from build123d import *

# Parameters (mm, degrees)
SKETCH_2_W               = 12.1
SKETCH_2_H               = 8
EXTRUDE_1_DEPTH          = 12.4
CUT_EXTRUDE_1_DEPTH      = 12.1
CUT_EXTRUDE_2_DEPTH      = 23.1
CUT_EXTRUDE_2_DEPTH_BACK = 16.1
HOLE_WIZARD_M31_D        = 3.4
HOLE_WIZARD_M31_DEPTH    = 10
HOLE_WIZARD_M31_TIP      = 1.021463052
FILLET_1_R               = 1


with BuildPart() as part:
    # Эскиз2 → Бобышка-Вытянуть1 (new body)
    with BuildSketch(Plane(origin=(0, 0, 0), x_dir=(0, 0, -1), z_dir=(1, 0, 0))):
        Polygon((-20.1, 10), (-20.1, 7), (0, 7), (0, 10), (15.1, 10), (15.1, -20), (12.1, -20), (12.1, 0), (0, 0), (0, -20), (-3, -20), (-3, 0), (-22.1, 0), (-22.1, 10), align=None)
        with Locations((6.05, -4)):
            Rectangle(SKETCH_2_W, SKETCH_2_H)
    extrude(amount=EXTRUDE_1_DEPTH)

    # Эскиз3 → Вырез-Вытянуть1 (cut)
    with BuildSketch(Plane.XY):
        with BuildLine():
            Line((0, 0), (-4.310236897, 0))
            Line((-4.310236897, 0), (-4.310236897, -10.158248203))
            Line((-4.310236897, -10.158248203), (16.784307367, -10.158248203))
            Line((16.784307367, -10.158248203), (16.784307367, 0))
            Line((16.784307367, 0), (12.4, 0))
            ThreePointArc((12.4, 0), (6.2, -6.2), (0, 0))
        make_face()
    extrude(amount=-CUT_EXTRUDE_1_DEPTH, mode=Mode.SUBTRACT)

    # Эскиз4 → Вырез-Вытянуть2 (cut, two sides)
    with BuildSketch(Plane.XY) as cut_extrude_2_sk:
        with BuildLine():
            Line((0, -13.8), (-4.529189241, -13.8))
            Line((-4.529189241, -13.8), (-4.529189241, -23.032738442))
            Line((-4.529189241, -23.032738442), (17.457291493, -23.032738442))
            Line((17.457291493, -23.032738442), (17.457291493, -13.8))
            Line((17.457291493, -13.8), (12.4, -13.8))
            ThreePointArc((12.4, -13.8), (6.2, -20), (0, -13.8))
        make_face()
    extrude(amount=CUT_EXTRUDE_2_DEPTH, mode=Mode.SUBTRACT)
    extrude(cut_extrude_2_sk.sketch, amount=-CUT_EXTRUDE_2_DEPTH_BACK, mode=Mode.SUBTRACT)

    # Отверстие с зазором M31
    with Locations(Plane(origin=(0, 7, 0), x_dir=(1, 0, 0), z_dir=(0, 1, 0))):
        with Locations((6.25, -10.05)):
            Hole(HOLE_WIZARD_M31_D / 2, depth=HOLE_WIZARD_M31_DEPTH)
            with Locations((0, 0, -(HOLE_WIZARD_M31_DEPTH + HOLE_WIZARD_M31_TIP / 2))):  # 118° drill point
                Cone(0, HOLE_WIZARD_M31_D / 2, HOLE_WIZARD_M31_TIP, mode=Mode.SUBTRACT)

    # Скругление1
    fillet_1_edges = [part.edges().sort_by_distance(p)[0] for p in [
        (6.2, 0, 22.1),
        (6.2, 10, 22.1),
    ]]
    fillet(fillet_1_edges, radius=FILLET_1_R)

    # Эскиз9 → Повернуть1 (revolve)
    with BuildSketch(Plane(origin=(6.2, 0, 0), x_dir=(0, 0, -1), z_dir=(1, 0, 0))):
        with BuildLine():
            Line((12.1, -20), (12.1, -18))
            Line((12.1, -18), (11.3, -18))
            ThreePointArc((11.3, -18), (11.507417596, -19.077032961), (12.1, -20))
        make_face()
    revolve(axis=Axis((6.2, -18, -11.3), (0, 0, -1)))


solid = part.part
The listing builds one solid part. Answer for the finished solid, in the listing's coordinates (mm). A direction names the side the tool comes from. Give positions to 0.01 mm unless a question says otherwise; leave off trailing zeros. Write each loop counter-clockwise with the first axis right and the second up, starting at its lowest first coordinate (ties: lowest second). Pieces come first, ordered by that corner, then holes. Notation, with made-up numbers: (78, 3) -> (121, 3) arc R23 cw to (121, 12) -> close; hole circle Ø11 at (-8, 8). An arc over 180 degrees is marked (long way). Use a Markdown table: item, result.
(1) Section B-B, the plane y = -7.5 is taken. Determine the outline of the cut face in (x, z), then the cut area to 3 significant figures.
Return value:
| item | result |
|---|---|
| outline | (0, -15.1) -> (12.4, -15.1) -> (12.4, -12.1) -> (0, -12.1) -> close; (0, 0) -> (12.4, 0) -> (12.4, 3) -> (0, 3) -> close |
| area | 74.4 mm2 |
(2) Section A-A, the plane z = 10.05 is taken. Determine the outline of the cut face in (x, y).
Return value:
| item | result |
|---|---|
| outline | (0, 0) -> (4.55, 0) -> (4.55, 7) -> (0, 7) -> close; (7.95, 0) -> (12.4, 0) -> (12.4, 7) -> (7.95, 7) -> close |
(3) Find the intervals of material crossed by probe 1 along X at (y, z) = (2.75, 10.05); probe 2 along Z at (x, y) = (10, -11.5); probe 3 along Z at (x, y) = (6.25, 4.25), in increasing order. Write a range as from..to.
Return value:
| item | result |
|---|---|
| probe 1 | 0..4.55, 7.95..12.4 |
| probe 2 | -15.1..-12.1, 0..3 |
| probe 3 | -15.1..8.35, 11.75..22.1 |
(4) Section C-C, the plane x = 5.5 is taken. Determine the outline of the cut face in (y, z), then the cut area to 3 significant figures.
Return value:
| item | result |
|---|---|
| outline | (-19.96, -15.1) -> (10, -15.1) -> (10, 0) -> (7, 0) -> (7, 8.52) -> (0, 8.52) -> (0, 3) -> (-19.96, 3) -> (-19.96, 0) -> (-6.16, 0) -> (-6.16, -12.1) -> (-16.13, -12.1) arc R2.81 ccw to (-19.87, -12.1) -> (-19.96, -12.1) -> close; (0, 11.58) -> (7, 11.58) -> (7, 20.1) -> (10, 20.1) -> (10, 21.1) arc R1 ccw to (9, 22.1) -> (1, 22.1) arc R1 ccw to (0, 21.1) -> close |
| area | 486 mm2 |
(5) For faces 1 (the flat face through (6, 0, 12)), 2 (the flat face through (12.4, 4, -1)), 3 (the flat face through (6, 7, 8)), determine the directions among +Z, -Z, +X, -X, +Y, -Y from which every point of the face is accessible in a straight line to the end or side of a thin tool.
Return value:
| item | result |
|---|---|
| face 1 | +Z, +X, -X, -Y |
| face 2 | +Z, -Z, +X, +Y, -Y |
| face 3 | +X, -X, +Y |
(6) Determine the mould class of faces 4 (the cylindrical face through (6.3, -20, -13.6)), 5 (the flat face through (6, 9, 20.1)), 6 (the flat face through (6, -12, -12.1)) for opening direction Y: released by +Y, released by -Y, zero draft, split by the parting line, or undercut.
Return value:
| item | result |
|---|---|
| face 4 | released by -Y |
| face 5 | zero draft |
| face 6 | undercut |
(7) Section D-D, the plane x = 9 is taken. Determine the outline of the cut face in (y, z), then the cut area to 3 significant figures.
Return value:
| item | result |
|---|---|
| outline | (-19.33, -15.1) -> (10, -15.1) -> (10, 0) -> (7, 0) -> (7, 20.1) -> (10, 20.1) -> (10, 21.1) arc R1 ccw to (9, 22.1) -> (1, 22.1) arc R1 ccw to (0, 21.1) -> (0, 3) -> (-19.33, 3) -> (-19.33, 0) -> (-5.53, 0) -> (-5.53, -12.1) -> (-19.33, -12.1) -> close |
| area | 494 mm2 |
(8) Flat-ended cylindrical pins translate along their axes: P1, Ø4, axis at x = 6.5, z = 7, coming from the +Y side; P2, Ø3, axis at x = 6.5, y = -8.5, coming from the +Z side; P3, Ø3, axis at x = 6, z = -6.5, coming from the -Y side. Find the tip coordinate at first contact, or state that the pin passes through.
Return value:
| item | result |
|---|---|
| P1 | y = 7 |
| P2 | z = 3 |
| P3 | y = -6.2 |
